Autodesk Inventor part; units mm, degrees
ref_plane "Płaszczyzna konstrukcyjna1" through (0, 5, 0) normal (0, -1, 0) x (1, 0, 0)
ref_plane "YZ Plane" through (0, 0, 0) normal (1, 0, 0) x (0, 1, 0)
ref_plane "XZ Plane" through (0, 0, 0) normal (0, 1, 0) x (-1, 0, 0)
sketch "Szkic1" plane through (0, 0, 0) normal (0, 1, 0) x (-1, 0, 0)
  line L0 (2.5, 6.1) -> (0, 6.1)
  line L1 (0, 6.1) -> (0, -6.1)
  line L2 (0, -6.1) -> (2.5, -6.1)
  line L3 (2.5, -6.1) -> (2.5, 6.1)
  line L4 (0, 6.1) -> (10, 6.1)
  line L5 (10, 6.1) -> (10, 4.6)
  line L6 (10, 4.6) -> (0, 4.6)
  line L7 (0, 4.6) -> (0, 6.1)
  line L8 (0, -4.6) -> (10, -4.6)
  line L9 (10, -4.6) -> (10, -6.1)
  line L10 (10, -6.1) -> (0, -6.1)
  line L11 (0, -6.1) -> (0, -4.6)
  point P0 (0, 0)
  point P1 (0, 0)
  point P2 (2.5, -6.1)
  point P3 (2.5, -4.6)
  point P4 (2.5, 4.6)
  dimension "d0" = 2.5
  dimension "d1" = 9.2
  dimension "d2" = 10
  dimension "d3" = 1.5
  dimension "d4" = 1.5
extrude "Wyciągnięcie proste1" add sketch "Szkic1" along normal blind 8
ref_plane "Płaszczyzna konstrukcyjna1" through (0, 5, 0) normal (0, -1, 0) x (1, 0, 0)
sketch "Szkic2" plane through (0, 5, 0) normal (0, -1, 0) x (1, 0, 0)
  line L0 (7, -4.45) -> (0, -4.45)
  line L1 (0, -4.45) -> (0, 4.45)
  line L2 (0, 4.45) -> (7, 4.45)
  line L3 (7, 4.45) -> (7, -4.45)
  point P0 (0, 0)
  point P1 (0, 0)
  dimension "d8" = 8.9
  dimension "d9" = 7
extrude "Wyciągnięcie proste2" add sketch "Szkic2" against normal blind 2.5
sketch "Szkic3" plane through (0, 7.5, 0) normal (0, 1, 0) x (1, 0, 0)
  line L0 (3.5, -4) -> (3.5, 4)
  line L1 (-13.4, 0) -> (10.4, 0)
  line L2 (7, 4.45) -> (0, 4.45)
  line L3 (0, -4.45) -> (7, -4.45)
  point P0 (0, 0)
  point P1 (3.5, 0)
  point P2 (0, 4.45)
  point P3 (3.5, -4.45)
  point P4 (3.5, 4.45)
hole "Otwór1" at (3.5, 7.5, 0) direction (0, -1, 0) diameter 2.6 end through all counterbore diameter 4.5 counterbore depth 1.5
fillet "Zaokrąglenie1" radius 2 2 edges at (7, 6.25, 4.45) (7, 6.25, -4.45)
fillet "Zaokrąglenie2" radius 1 4 edges at (-10, 4, -6.1) (0, 4, -6.1) (-10, 4, 6.1) (0, 4, 6.1)
equation "\"d0\" = holder_gniazdo_grubosc"
equation "\"d1\" = holder_gniazdo_odleglosc_miedzy_ramionami"
equation "\"d2\" = holder_gniazdo_dlugosc_ramion"
equation "\"d3\" = holder_gniazdo_grubosc_ramion"
equation "\"d4\" = holder_gniazdo_grubosc_ramion"
equation "\"d5\" = holder_gniazdo_wys"
equation "\"d8\" = podstawa_mocowanie_DC_b"
equation "\"d9\" = podstawa_mocowanie_DC_a"
equation "\"d10\" = holder_gniazdo_grubosc"
equation "\"d12\" = gniazdo_M2_D2"
equation "\"d14\" = gniazdo_M2_D1"
equation "\"d15\" = gniazdo_M2_glebokosc"
equation "\"gniazdo_M2_glebokosc\" = 1.5"
equation "\"gniazdo_M2_D1\" = 4.5"
equation "\"gniazdo_M2_D2\" = 2.6"
equation "\"insert_D\" = 2.9"
equation "\"insert_glebokosc\" = 7"
equation "\"podstawa_wys\" = 2"
equation "\"podstawa_otwory_montazowe_poz_x\" = 4"
equation "\"podstawa_otwory_montazowe_poz_y\" = 4"
equation "\"podstawa_zaokraglenie\" = 3"
equation "\"obudowa_wys\" = 45"
equation "\"obudowa_grubosc\" = 2"
equation "\"obudowa_kontrolki_a\" = 38"
equation "\"obudowa_otwory_montazowe_poz_x\" = 4"
equation "\"obudowa_otwory_montazowe_poz_y\" = 4"
equation "\"obudowa_otwory_montazowe_material_x\" = 8"
equation "\"obudowa_otwory_montazowe_material_y\" = 8"
equation "\"obudowa_zaokraglenie\" = 3"
equation "\"obudowa_otwory_io1_D\" = 12"
equation "\"obudowa_otwory_io1_wys\" = 25"
equation "\"obudowa_otwory_io1_poz\" = 55"
equation "\"obudowa_otwory_io2_D\" = 12"
equation "\"obudowa_otwory_io2_wys\" = 25"
equation "\"obudowa_otwory_io2_poz\" = 38"
equation "\"obudowa_otwory_pot_D\" = 7.2"
equation "\"obudowa_pot_poz_y\" = 15"
equation "\"obudowa_s_rozstaw_y\" = 16"
equation "\"obudowa_s_poz_x\" = 78"
equation "\"obudowa_s_poz_y\" = 15"
equation "\"obudowa_s_D\" = 6.2"
equation "\"input_a\" = 8.9"
equation "\"input_b\" = 14.4"
equation "\"input_wys\" = 10.9"
equation "\"obudowa_MTS_otwor_D\" = 6.2"
equation "\"pcb_rozstaw_x\" = 92"
equation "\"pcb_rozstaw_y\" = 58"
equation "\"pcb_grubosc_scianki\" = 6"
equation "\"pcb_wys_bloku\" = 35"
equation "\"pcb_poz_y\" = 29"
equation "\"obudowa_footswitch_D\" = 12.3"
equation "\"obudowa_footswitch_poz_x\" = 35"
equation "\"obudowa_footswitch_poz_y\" = 68"
equation "\"obudowa_led_indicator_D\" = 3.5"
equation "\"obudowa_led_indicator_poz_x\" = 55"
equation "\"obudowa_podkladka_otwory\" = 4"
equation "\"obudowa_uchwyt_poz_z\" = 3"
equation "\"obudowa_uchwyt_grubosc\" = 2"
equation "\"obudowa_uchwyt_szerokosc_wew\" = 17.5"
equation "\"obudowa_uchwyt_wysokosc_wew\" = 26.3"
equation "\"obudowa_uchwyt_kolnierz_wys\" = 55"
equation "\"obudowa_gniazdo_poz\" = 25"
equation "\"obudowa_podciecie_inout_wys\" = 6"
equation "\"obudowa_podciecie_logo_wys\" = 34"
equation "\"obudowa_podciecie_logo_szerokosc\" = 25"
equation "\"obudowa_pot_pozycjonowanie_szerokosc\" = 2.8"
equation "\"obudowa_pot_pozycjonowanie_wys\" = 13"
equation "\"obudowa_pot_pozycjonowanie_glebokosc\" = 1.4"
equation "\"obudowa_led_mocowanie_wys\" = 6"
equation "\"obudowa_led_mocowanie_grubosc\" = 8"
equation "\"holder_led_grubosc\" = 2.5"
equation "\"holder_led_dlugosc\" = 28"
equation "\"holder_led_uchwyt_D\" = 5"
equation "\"holder_led_uchwyt_szerokosc\" = 8"
equation "\"holder_led_uchwyt_wysokosc\" = 5"
equation "\"holder_gniazdo_grubosc\" = 2.5"
equation "\"holder_gniazdo_a\" = 28"
equation "\"holder_gniazdo_b\" = 5"
equation "\"podstawa_mocowanie_DC_a\" = 7"
equation "\"podstawa_mocowanie_DC_b\" = 8.9"
equation "\"podstawa_mocowanie_DC_wys\" = 6"
equation "\"holder_gniazdo_odleglosc_miedzy_ramionami\" = 9.2"
equation "\"holder_gniazdo_dlugosc_ramion\" = 10"
equation "\"holder_gniazdo_grubosc_ramion\" = 1.5"
equation "\"holder_gniazdo_wys\" = 8"
equation "\"holder_gniazdo_uchwyt_poz\" = 5"
equation "\"d7\" = -holder_gniazdo_uchwyt_poz"
properties part number "input_holder"
Source: CAD feature listing. Evaluate the final solid. Frame: model axes, mm. A direction names the side the tool comes from. Give positions to 0.01 mm unless a question says otherwise; leave off trailing zeros. Order: outer loops, then holes, each group sorted by start corner. A loop starts at its lowest first (then second) coordinate and runs counter-clockwise, first axis right, second up. Notation, with made-up numbers: (21, -16.75) -> (52, -16.75) arc R21 ccw to (52, 17.25) -> close; hole circle Ø8 at (71, -39). An arc over 180 degrees is marked (long way). Write item = value, one per line.
Q1. Set-up query: faces 1 (the face through (-2, 0, 0)), 2 (the face through (5.496, 6.74, 1.038)), 3 (the face through (-6, 4, 4.6)), 4 (the face through (2, 5, 0)), 5 (the face through (-0.285, 4.056, -5.799)). Return all of +Z, -Z, +X, -X, +Y, -Y with unobstructed straight access to the full face (end or side cutting, diameter ignored); none if empty.
Data:
face_1 = +Z, -Z, +X, -X, -Y
face_2 = +Y
face_3 = -X, +Y, -Y
face_4 = +Z, -Z, +X, -Y
face_5 = -Z, +X, +Y, -Y
Q2. Material intervals for line 1 (X direction, y = 5.6, z = 0); line 2 (Z direction, x = 3.5, y = 5.6); line 3 (X direction, y = 6.45, z = 0), sorted ascending. Write a range as from..to.
Data:
line_1 = -2.5..2.2, 4.8..7
line_2 = -4.45..-1.3, 1.3..4.45
line_3 = -2.5..1.25, 5.75..7
Q3. Cut plane B-B, the plane z = 0. Output: boundary loops of the cut face in (x, y).
Data:
outline = (-2.5, 0) -> (0, 0) -> (0, 5) -> (2.2, 5) -> (2.2, 6) -> (1.25, 6) -> (1.25, 7.5) -> (0, 7.5) -> (0, 8) -> (-2.5, 8) -> close; (4.8, 5) -> (7, 5) -> (7, 7.5) -> (5.75, 7.5) -> (5.75, 6) -> (4.8, 6) -> close
Q4. Pin query (flat end, axial travel): pin 1 (2 mm diameter, centred on x = 1.5, y = 6, fed in from -Z); pin 2 (2 mm diameter, centred on y = 6, z = 3.5, fed in from -X); pin 3 (3.5 mm diameter, centred on x = 4, z = -0.5, fed in from +Y). Return the tip coordinate at first contact, or that it passes through.
Data:
pin_1 = -4.45
pin_2 = -2.5
pin_3 = 7.5
Q5. Cut plane D-D, the plane y = 4.5. Output: boundary loops of the cut face in (x, z), and give its area (3 significant figures).
Data:
outline = (-10, -5.1) arc R1 ccw to (-9, -6.1) -> (-1, -6.1) arc R1 ccw to (0, -5.1) -> (0, 5.1) arc R1 ccw to (-1, 6.1) -> (-9, 6.1) arc R1 ccw to (-10, 5.1) -> (-10, 4.6) -> (-2.5, 4.6) -> (-2.5, -4.6) -> (-10, -4.6) -> close
area = 52.1 mm^2
Q6. Cut plane A-A, the plane x = 3.5. Output: boundary loops of the cut face in (y, z).
Data:
outline = (5, -4.45) -> (7.5, -4.45) -> (7.5, -2.25) -> (6, -2.25) -> (6, -1.3) -> (5, -1.3) -> close; (5, 1.3) -> (6, 1.3) -> (6, 2.25) -> (7.5, 2.25) -> (7.5, 4.45) -> (5, 4.45) -> close
Q7. Cut plane C-C, the plane y = 7. Output: boundary loops of the cut face in (x, z).
Data:
outline = (-10, -5.1) arc R1 ccw to (-9, -6.1) -> (-1, -6.1) arc R1 ccw to (0, -5.1) -> (0, -4.45) -> (5, -4.45) arc R2 ccw to (7, -2.45) -> (7, 2.45) arc R2 ccw to (5, 4.45) -> (0, 4.45) -> (0, 5.1) arc R1 ccw to (-1, 6.1) -> (-9, 6.1) arc R1 ccw to (-10, 5.1) -> (-10, 4.6) -> (-2.5, 4.6) -> (-2.5, -4.6) -> (-10, -4.6) -> close; hole circle Ø4.5 at (3.5, 0)
Q8. Pull-direction query (Z, two-part tool) for faces 6 (the face through (6.43, 6.27, -3.85)), 7 (the face through (-0.301, 4.056, 5.815)), 8 (the face through (-2.5, 4, 0)); classes: released by +Z, released by -Z, zero draft, split by the parting line, or undercut.
Data:
face_6 = released by -Z
face_7 = released by +Z
face_8 = undercut
